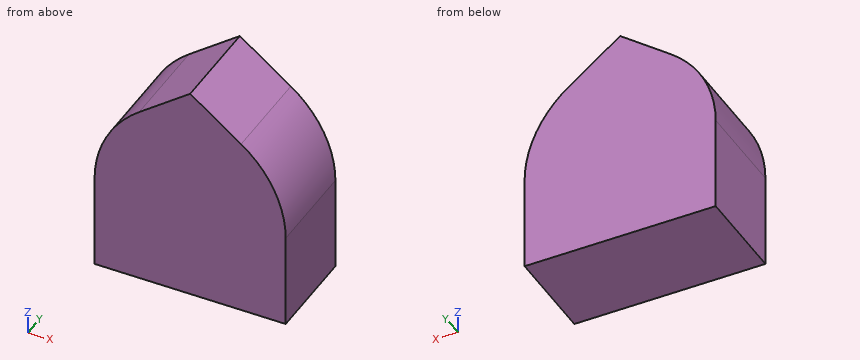
from build123d import *

# Parameters (mm, degrees)
F1_DEPTH = 152.4


with BuildPart() as f1:
    # F0 (on Front) → F1 (new body)
    with BuildSketch(Plane.XZ):
        with BuildLine():
            Line((-152.4, 152.4), (-152.4, 0))
            Line((-152.4, 0), (152.4, 0))
            Line((152.4, 0), (152.4, 152.4))
            ThreePointArc((152.4, 152.4), (133.629155, 231.914577), (81.28, 294.64))
            Line((81.28, 294.64), (0, 355.6))
            Line((0, 355.6), (-81.28, 294.64))
            ThreePointArc((-81.28, 294.64), (-133.629155, 231.914577), (-152.4, 152.4))
        make_face()
    extrude(amount=F1_DEPTH)


solid = f1.part
Part model, mm, in its own coordinate system. Give positions to 0.01 mm unless a question says otherwise; leave off trailing zeros. Write each loop counter-clockwise with the first axis right and the second up, starting at its lowest first coordinate (ties: lowest second). Pieces come first, ordered by that corner, then holes.
1) Cut at A-A on y = -96. Write the cut outline in (x, z).
Resolved:
outline: (-152.4, 0) - (152.4, 0) - (152.4, 152.4) arc R177.8 ccw to (81.28, 294.64) - (0, 355.6) - (-81.28, 294.64) arc R177.8 ccw to (-152.4, 152.4) - close
2) Probe L1, parallel to Z at x = 105.5, y = -128.5; L2, parallel to Z at x = 90.5, y = -8.5; L3, parallel to X at y = -64.5, z = 163. List the from-to ranges inside material, lowest first.
Resolved:
L1: z = 0 to 272.72
L2: z = 0 to 287.23
L3: x = -152.08 to 152.08
3) Cut at B-B on x = -75. Write the cut outline in (y, z), then the cut area to 3 significant figures.
Resolved:
outline: (-152.4, 0) - (0, 0) - (0, 299.35) - (-152.4, 299.35) - close
area: 45,600 mm2
4) Pin check, flat tips, straight feed: pin 1 (2 mm diameter, centred on y = -89, z = 210.5, fed in from +X); pin 2 (2 mm diameter, centred on y = -109.5, z = 256, fed in from -X); pin 3 (6 mm diameter, centred on y = -67, z = 191, fed in from +X). Stop position of each tip, or through.
Resolved:
pin 1: stops at x = 142.98
pin 2: stops at x = -119.81
pin 3: stops at x = 148.8
5) Cut at C-C on z = 323. Write the cut outline in (x, y), then the cut area to 3 significant figures.
Resolved:
outline: (-43.47, -152.4) - (43.47, -152.4) - (43.47, 0) - (-43.47, 0) - close
area: 13,200 mm2
